CAD build for the part. Positions are in the model's coordinates, mm. Face numbers are marked on the shaded views. A direction names the side the tool comes from. Round coordinates to 2 decimals unless told otherwise and drop trailing zeros. Write each loop counter-clockwise with the first axis right and the second up, starting at its lowest first coordinate (ties: lowest second). Pieces come first, ordered by that corner, then holes. Notation, with made-up numbers: (-21, 50) -> (28, 50) arc R16 ccw to (28, 55) -> close; hole circle Ø6 at (42, 26.5). An arc over 180 degrees is marked (long way). Put each result on its own line as item: value. Start each with the question number.
1. Saw through at B-B on x = 16. List the corners of the cut face in (y, z), and give its area (3 significant figures).
2. Saw through at D-D on z = 7.5. List the corners of the cut face in (x, y), and give its area (3 significant figures).
3. Saw through at C-C on z = 20.5. State how many separate pieces and enclosed holes the cut face has, and give its area (3 significant figures).
4. 3-axis set-ups, long thin cutter, end or side, ignore diameter. For the marked faces 1, 2 and 3: which of +Z, -Z, +X, -X, +Y, -Y reach the whole face in a straight line?
5. Flat gauge pins, fed straight in: P1, Ø2.5, axis at y = -2, z = 19.5, coming from the -X side; P2, Ø4.5, axis at x = 16.5, z = 6, coming from the +Y side; P3, Ø1.5, axis at y = -2, z = 7, coming from the +X side. Where does each tip first touch, or does it go through?
6. Saw through at A-A on y = -0.5. List the corners of the cut face in (x, z).
7. Drill centre lines: line 1 (Z direction, x = -16, y = -5.9); line 2 (Z direction, x = 16, y = -7.1); line 3 (X direction, y = -2, z = 7). Where is each one in solid material? Low to high. Write a range as from..to.
8. Pull direction X, two halves, no side cores. Call the marked faces 4, 5, 6 and 7: pulls with the +X half, pulls with the -X half, needs draft (parallel to the pull), parting line crosses it, or undercut.
from build123d import *

# Parameters (mm, degrees)
SKETCH3_W           = 14.8
SKETCH3_H           = 2.7
BOSS_EXTRUDE3_DEPTH = 26
SKETCH4_R           = 1.05
CUT_EXTRUDE1_DEPTH  = 40.141282554
SKETCH5_R           = 2
CUT_EXTRUDE2_DEPTH  = 1.9
FILLET2_R           = 2


with BuildPart() as part:
    # Sketch3 → Boss-Extrude3 (new body)
    with BuildSketch(Plane.XY):
        with BuildLine():
            ThreePointArc((10.2, 0), (0, 10.2), (-10.2, 0))
            ThreePointArc((-10.2, 0), (-9.867181258, -2.584324675), (-8.890444308, -5))
            Line((-8.890444308, -5), (-8.2, -5))
            Line((-8.2, -5), (-8.2, 0))
            ThreePointArc((-8.2, 0), (0, 8.2), (8.2, 0))
            Line((8.2, 0), (8.2, -5))
            Line((8.2, -5), (8.890444308, -5))
            ThreePointArc((8.890444308, -5), (9.867181258, -2.584324675), (10.2, 0))
        make_face()
        with BuildLine():
            Line((-10.2, 0), (-10.2, -5))
            Line((-10.2, -5), (-8.890444308, -5))
            ThreePointArc((-8.890444308, -5), (-9.867181258, -2.584324675), (-10.2, 0))
        make_face()
        with BuildLine():
            ThreePointArc((-8.890444308, -5), (-8.561838049, -5.543909201), (-8.2, -6.066300355))
            Line((-8.2, -6.066300355), (-8.2, -5))
            Line((-8.2, -5), (-8.890444308, -5))
        make_face()
        with BuildLine():
            Line((-10.2, -5), (-10.2, -7.7))
            Line((-10.2, -7.7), (-8.2, -7.7))
            Line((-8.2, -7.7), (-8.2, -6.066300355))
            ThreePointArc((-8.2, -6.066300355), (-8.561838049, -5.543909201), (-8.890444308, -5))
            Line((-8.890444308, -5), (-10.2, -5))
        make_face()
        with Locations((-17.6, -6.35)):
            Rectangle(SKETCH3_W, SKETCH3_H)
        with BuildLine():
            Line((10.2, -5), (10.2, 0))
            ThreePointArc((10.2, 0), (9.867181258, -2.584324675), (8.890444308, -5))
            Line((8.890444308, -5), (10.2, -5))
        make_face()
        with BuildLine():
            Line((8.2, -5), (8.2, -6.066300355))
            ThreePointArc((8.2, -6.066300355), (8.561838049, -5.543909201), (8.890444308, -5))
            Line((8.890444308, -5), (8.2, -5))
        make_face()
        with BuildLine():
            Line((8.2, -6.066300355), (8.2, -7.7))
            Line((8.2, -7.7), (10.2, -7.7))
            Line((10.2, -7.7), (10.2, -5))
            Line((10.2, -5), (8.890444308, -5))
            ThreePointArc((8.890444308, -5), (8.561838049, -5.543909201), (8.2, -6.066300355))
        make_face()
        with Locations((17.6, -6.35)):
            Rectangle(SKETCH3_W, SKETCH3_H)
    extrude(amount=BOSS_EXTRUDE3_DEPTH)

    # Sketch4 → Cut-Extrude1 (cut, through all)
    with BuildSketch(Plane(origin=(0, -5, 0), x_dir=(1, 0, 0), z_dir=(0, 1, 0))):
        with Locations(Location((-16, -5.022119535, 0), (0, 0, 180))):
            Circle(SKETCH4_R)
        with Locations(Location((-16, -21.022119535, 0), (0, 0, 180))):
            Circle(SKETCH4_R)
        with Locations(Location((16, -5.022119535, 0), (0, 0, 180))):
            Circle(SKETCH4_R)
        with Locations(Location((16, -21.022119535, 0), (0, 0, 180))):
            Circle(SKETCH4_R)
    extrude(amount=-CUT_EXTRUDE1_DEPTH, mode=Mode.SUBTRACT)

    # Sketch5 → Cut-Extrude2 (cut)
    with BuildSketch(Plane(origin=(0, -5, 0), x_dir=(1, 0, 0), z_dir=(0, 1, 0))):
        with Locations(Location((-16, -5.022119535, 0), (0, 0, 180))):
            Circle(SKETCH5_R)
        with Locations(Location((16, -5.022119535, 0), (0, 0, 180))):
            Circle(SKETCH5_R)
        with Locations(Location((16, -21.022119535, 0), (0, 0, 180))):
            Circle(SKETCH5_R)
        with Locations(Location((-16, -21.022119535, 0), (0, 0, 180))):
            Circle(SKETCH5_R)
    extrude(amount=-CUT_EXTRUDE2_DEPTH, mode=Mode.SUBTRACT)

    # Fillet2
    fillet2_edges = [part.edges().sort_by_distance(p)[0] for p in [
        (8.2, -7.7, 13),
        (-8.2, -7.7, 13),
    ]]
    fillet(fillet2_edges, radius=FILLET2_R)


solid = part.part
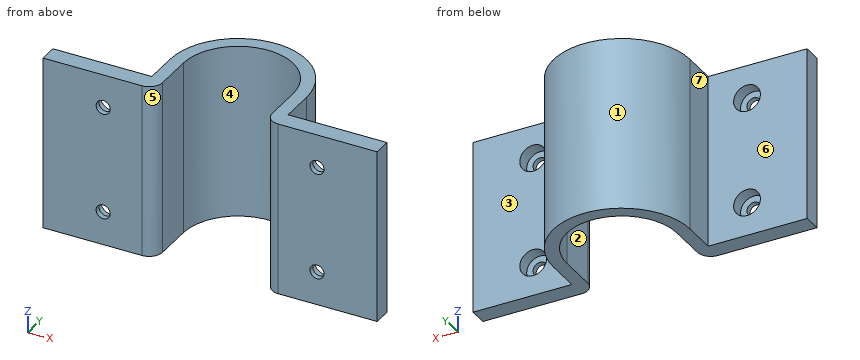
Return value:
1. outline: (-7.7, 0) -> (-5, 0) -> (-5, 3.02) -> (-6.9, 3.02) -> (-6.9, 3.97) -> (-7.7, 3.97) -> close; (-7.7, 6.07) -> (-6.9, 6.07) -> (-6.9, 7.02) -> (-5, 7.02) -> (-5, 19.02) -> (-6.9, 19.02) -> (-6.9, 19.97) -> (-7.7, 19.97) -> close; (-7.7, 22.07) -> (-6.9, 22.07) -> (-6.9, 23.02) -> (-5, 23.02) -> (-5, 26) -> (-7.7, 26) -> close
1. area: 51.6 mm^2
2. outline: (-25, -7.7) -> (-10.2, -7.7) arc R2 ccw to (-8.2, -5.7) -> (-8.2, 0) arc R8.2 cw to (8.2, 0) -> (8.2, -5.7) arc R2 ccw to (10.2, -7.7) -> (25, -7.7) -> (25, -5) -> (10.2, -5) -> (10.2, 0) arc R10.2 ccw to (-10.2, 0) -> (-10.2, -5) -> (-25, -5) -> close
2. area: 167 mm^2
3. separate pieces: 3
3. enclosed holes: 0
3. area: 149 mm^2
4. face 1: +Z, -Z, +Y
4. face 2: +Z, -Z, -Y
4. face 3: +Z, -Z, +X, +Y
5. P1: stops at x = -10.2
5. P2: stops at y = -5
5. P3: stops at x = 10.2
6. outline: (-10.2, 0) -> (-8.2, 0) -> (-8.2, 26) -> (-10.2, 26) -> close; (8.2, 0) -> (10.2, 0) -> (10.2, 26) -> (8.2, 26) -> close
7. line 1: z = 0..3.02, 7.02..19.02, 23.02..26
7. line 2: z = 0..3.97, 6.07..19.97, 22.07..26
7. line 3: x = -10.2..-8.2, 8.2..10.2
8. face 4: undercut
8. face 5: undercut
8. face 6: needs draft
8. face 7: pulls with the -X half
